Build history of the part. All positions in model axes, mm. A direction names the side the tool comes from. Round coordinates to 2 decimals unless told otherwise and drop trailing zeros. Order: outer loops, then holes, each group sorted by start corner. A loop starts at its lowest first (then second) coordinate and runs counter-clockwise, first axis right, second up. Notation, with made-up numbers: (85.5, 3) -> (133.5, 3) arc R15 ccw to (133.5, 19) -> close; hole circle Ø8 at (83.5, -35). An arc over 180 degrees is marked (long way). Write item = value, one per line.
from build123d import *

# Parameters (mm, degrees)
F0_W     = 20
F0_H     = 30
F1_DEPTH = 10
F2_W     = 20
F2_H     = 30
F3_DEPTH = 5
F4_SIZE  = 7


with BuildPart() as f1:
    # F0 (on Top) → F1 (new body)
    with BuildSketch(Plane.XY):
        Rectangle(F0_W, F0_H)
        with BuildLine():
            ThreePointArc((2.25, -10), (-1.5909902577, -11.5909902577), (0, -7.75))
            ThreePointArc((0, -7.75), (1.5909902577, -8.4090097423), (2.25, -10))
        make_face(mode=Mode.SUBTRACT)
        with BuildLine():
            ThreePointArc((0, -6.75), (-2.25, -4.5), (0, -2.25))
            ThreePointArc((0, -2.25), (1.5909902577, -2.9090097423), (2.25, -4.5))
            ThreePointArc((2.25, -4.5), (1.5909902577, -6.0909902577), (0, -6.75))
        make_face(mode=Mode.SUBTRACT)
        with BuildLine():
            ThreePointArc((2.25, 4.5), (1.5909902577, 2.9090097423), (0, 2.25))
            ThreePointArc((0, 2.25), (-2.25, 4.5), (0, 6.75))
            ThreePointArc((0, 6.75), (1.5909902577, 6.0909902577), (2.25, 4.5))
        make_face(mode=Mode.SUBTRACT)
        with BuildLine():
            ThreePointArc((2.25, 10), (1.5909902577, 8.4090097423), (0, 7.75))
            ThreePointArc((0, 7.75), (-1.5909902577, 11.5909902577), (2.25, 10))
        make_face(mode=Mode.SUBTRACT)
    extrude(amount=F1_DEPTH)

    # F2 (on face) → F3 (join)
    with BuildSketch(Plane.XY.offset(10)):
        Rectangle(F2_W, F2_H)
        with BuildLine():
            ThreePointArc((2.25, -10), (-1.5909902577, -11.5909902577), (0, -7.75))
            ThreePointArc((0, -7.75), (1.5909902577, -8.4090097423), (2.25, -10))
        make_face(mode=Mode.SUBTRACT)
        Polygon((0, 7.6447422616), (6.1318632215, 7.6447422616), (6.1318632215, -7.6447422616), (0, -7.6447422616), (-6.1318632215, -7.6447422616), (-6.1318632215, 7.6447422616), align=None, mode=Mode.SUBTRACT)
        with BuildLine():
            ThreePointArc((2.25, 10), (1.5909902577, 8.4090097423), (0, 7.75))
            ThreePointArc((0, 7.75), (-1.5909902577, 11.5909902577), (2.25, 10))
        make_face(mode=Mode.SUBTRACT)
    extrude(amount=F3_DEPTH)

    # F4
    f4_edges = [f1.edges().sort_by_distance(p)[0] for p in [
        (-10, 15, 7.5),
        (-10, -15, 7.5),
        (10, 15, 7.5),
        (10, -15, 7.5),
    ]]
    chamfer(f4_edges, length=F4_SIZE)


solid = f1.part
Q1. Cut at C-C, the plane x = -5.25. List the corners of the cut face in (y, z).
Check values:
outline = (-12.75, 0) -> (12.75, 0) -> (12.75, 15) -> (7.64, 15) -> (7.64, 10) -> (-7.64, 10) -> (-7.64, 15) -> (-12.75, 15) -> close
Q2. Cut at D-D, the plane z = 13.5. List the corners of the cut face in (x, y), and give its area (3 significant figures).
Check values:
outline = (-10, -8) -> (-3, -15) -> (3, -15) -> (10, -8) -> (10, 8) -> (3, 15) -> (-3, 15) -> (-10, 8) -> close; hole (-6.13, -7.64) -> (6.13, -7.64) -> (6.13, 7.64) -> (-6.13, 7.64) -> close; hole circle Ø4.5 at (0, -10); hole circle Ø4.5 at (0, 10)
area = 283 mm²
Q3. Cut at A-A, the plane y = -10. List the corners of the cut face in (x, z), and give its area (4 significant figures).
Check values:
outline = (-8, 0) -> (-2.25, 0) -> (-2.25, 15) -> (-8, 15) -> close; (2.25, 0) -> (8, 0) -> (8, 15) -> (2.25, 15) -> close
area = 172.5 mm²
Q4. Mould opens along Y. For faces 3 (the face through (10, 0, 7)), 4 (the face through (1, 7.645, 12)), 5 (the face through (7, -11, 7)), 6 (the face through (-6, 12, 8)) say: released by +Y, released by -Y, zero draft, split by the parting line, or undercut.
Check values:
face_3 = zero draft
face_4 = undercut
face_5 = released by -Y
face_6 = released by +Y
Q5. Cut at B-B, the plane z = 3.5. List the corners of the cut face in (x, y).
Check values:
outline = (-10, -8) -> (-3, -15) -> (3, -15) -> (10, -8) -> (10, 8) -> (3, 15) -> (-3, 15) -> (-10, 8) -> close; hole circle Ø4.5 at (0, -10); hole circle Ø4.5 at (0, -4.5); hole circle Ø4.5 at (0, 4.5); hole circle Ø4.5 at (0, 10)
Q6. Flat gauge pins, fed straight in: pin 1 (1 mm diameter, centred on x = -7.5, z = 6, fed in from -Y); pin 2 (10 mm diameter, centred on x = 2.5, y = 3, fed in from +Z); pin 3 (3.5 mm diameter, centred on x = 0, y = 10, fed in from -Z); pin 4 (1.5 mm diameter, centred on y = -12, z = 10, fed in from +X). Where does each tip first touch, or does it go through?
Check values:
pin_1 = -11
pin_2 = 15
pin_3 = through
pin_4 = 6.75
Q7. Probe probe 1 along Y at (x, z) = (-0.75, 3.25); probe 2 along X at (y, z) = (-10, 5.5); probe 3 along X at (y, z) = (-2.5, 11.25). List the from-to ranges inside material, lowest first.
Check values:
probe_1 = -15 to -12.12, -7.88 to -6.62, -2.38 to 2.38, 6.62 to 7.88, 12.12 to 15
probe_2 = -8 to -2.25, 2.25 to 8
probe_3 = -10 to -6.13, 6.13 to 10
Q8. Which spindle directions (+Z, -Z, +X, -X, +Y, -Y) get a long thin tool onto all of the face, cutting with end or side? Do faces 1 (the face through (0, 0, 10)), 2 (the face through (2.08, 10.86, 7.4)). Say none if no direction does.
Check values:
face_1 = +Z
face_2 = +Z, -Z
